The listing builds one solid part. Answer for the finished solid, in the listing's coordinates (mm). A direction names the side the tool comes from. Give positions to 0.01 mm unless a question says otherwise; leave off trailing zeros. Order: outer loops, then holes, each group sorted by start corner. A loop starts at its lowest first (then second) coordinate and runs counter-clockwise, first axis right, second up. Notation, with made-up numbers: (-15.5, -26) -> (-2.5, -26) arc R29 cw to (-2.5, -3) -> close; hole circle Ø9 at (64.5, 48). An arc over 180 degrees is marked (long way). One line per question, with ' | ' between items. Start each with the question number.
Autodesk Inventor part; units mm, degrees
ref_plane "YZ Plane" through (0, 0, 0) normal (1, 0, 0) x (0, 1, 0)
ref_plane "XZ Plane" through (0, 0, 0) normal (0, 1, 0) x (-1, 0, 0)
ref_plane "XY Plane" through (0, 0, 0) normal (0, 0, 1) x (1, 0, 0)
sketch "Esquisse1" plane through (0, 0, 0) normal (0, 1, 0) x (-1, 0, 0)
  circle A0 centre (0, 0) radius 9
  dimension "d0" = 18
extrude "Extrusion1" add sketch "Esquisse1" along normal blind 1
sketch "Esquisse2" plane through (0, 1, 0) normal (0, 1, 0) x (1, 0, 0)
  circle A0 centre (0, 0) radius 9
  circle A1 centre (0, 0) radius 4
  dimension "d3" = 8
extrude "Extrusion2" add sketch "Esquisse2" along normal blind 13 contours A1
sketch "Esquisse3" plane through (0, 14, 0) normal (0, 1, 0) x (1, 0, 0)
  circle A0 centre (0, 0) radius 4
  arc A1 (-2.25, 1.0897) -> (2.25, 1.0897) centre (0, 0) ccw
  line L0 (-2.25, 1.0897) -> (2.25, 1.0897)
  arc A2 (2.25, 1.0897) -> (-2.25, 1.0897) centre (0, 0) ccw
  dimension "d6" = 5
  dimension "d10" = 4.5
extrude "Extrusion3" cut sketch "Esquisse3" against normal through all contours L0 A1
sketch "Esquisse4" plane through (-2.25, 14, -1.0897) normal (0, 0, 1) x (1, 0, 0)
  line L0 (0, 0) -> (4.5, 0)
  line L1 (2.25, -14) -> (2.25, 0) construction
  circle A0 centre (2.25, -10) radius 1.5
  dimension "d11" = 4
  dimension "d12" = 3
extrude "Extrusion4" cut sketch "Esquisse4" against normal up to next
sketch "Esquisse5" plane through (0, 1, 0) normal (0, 1, 0) x (1, 0, 0)
  circle A0 centre (0, 0) radius 4
  circle A1 centre (0, 0) radius 9
  line L0 (0, 0) -> (0, 9) construction
  circle A2 centre (0, 6.5) radius 1.2128
  dimension "d15" = 2.4255
  dimension "d16" = 6.5
extrude "Extrusion5" cut sketch "Esquisse5" against normal up to next contours A2
pattern_circular "Réseau circulaire1" count 6 over 360 about axis through (0, -10, 0) along (0, 1, 0) of "Extrusion5"
thread "Filetage1"
properties part number "axe_roue_moteur"
(1) The part is cut by section A-A on z = 0. Determine the outline of the cut face in (x, y), plus the area to 3 significant figures.
(2) Given P1, Ø3, axis at x = 2, y = 3.5, coming from the -Z side; P2, Ø4, axis at y = 8.5, z = -1.5, coming from the -X side; P3, Ø4, axis at y = 9.5, z = 3, coming from the -X side; P4, Ø1.5, axis at x = -5.63, z = 3.25, coming from the +Y side, each flat-ended and moving along its own axis, determine where each tip first touches the part or whether it passes through.
(3) The part is cut by section D-D on x = 6. Determine the outline of the cut face in (y, z).
(4) For faces 1 (the face through (-1.5, 4.07, -2.52)), 2 (the face through (0, 7, -1.09)), 3 (the face through (-2, 1, -4)), determine the directions among +Z, -Z, +X, -X, +Y, -Y from which every point of the face is accessible in a straight line to the end or side of a thin tool.
(5) The part is cut by section B-B on z = -3.25. Determine the outline of the cut face in (x, y), plus the area to 3 significant figures.
(6) Consider line 1 (Z direction, x = 0, y = 0.5); line 2 (Z direction, x = 0, y = 8); line 3 (Y direction, x = 4.25, z = 7). Determine where each line is inside the solid, lowest interval first.
(7) Determine the mould class of faces 4 (the face through (2.15, 7.409, 3.373)), 5 (the face through (0.263, 0.507, 5.316)), 6 (the face through (0, 14, -2)) for opening direction Z: pulls with the +Z half, pulls with the -Z half, needs draft (parallel to the pull), parting line crosses it, or undercut.
(8) The part is cut by section C-C on z = 3.25. Determine the outline of the cut face in (x, y).
Result sheet:
1) outline: (-9, 0) -> (-2.5, 0) -> (-2.5, 14) -> (-4, 14) -> (-4, 1) -> (-9, 1) -> close; (2.5, 0) -> (9, 0) -> (9, 1) -> (4, 1) -> (4, 14) -> (2.5, 14) -> close | area: 52.0 mm^2
2) P1: stops at z = -3.93 | P2: stops at x = -4 | P3: stops at x = -3.87 | P4: passes through
3) outline: (0, -6.71) -> (1, -6.71) -> (1, -4.4) -> (0, -4.4) -> close; (0, -2.1) -> (1, -2.1) -> (1, 2.1) -> (0, 2.1) -> close; (0, 4.4) -> (1, 4.4) -> (1, 6.71) -> (0, 6.71) -> close
4) face 1: -Z | face 2: +Y, -Y | face 3: +Y
5) outline: (-8.39, 0) -> (-6.84, 0) -> (-6.84, 1) -> (-8.39, 1) -> close; (-4.42, 0) -> (4.42, 0) -> (4.42, 1) -> (2.33, 1) -> (2.33, 14) -> (-2.33, 14) -> (-2.33, 1) -> (-4.42, 1) -> close; (6.84, 0) -> (8.39, 0) -> (8.39, 1) -> (6.84, 1) -> close; hole circle Ø3 at (0, 4) | area: 65.5 mm^2
6) line 1: z = -9 to -7.71, -5.29 to -1.09, 2.5 to 5.29, 7.71 to 9 | line 2: z = -4 to -1.09, 2.5 to 4 | line 3: y = 0 to 1
7) face 4: parting line crosses it | face 5: undercut | face 6: needs draft
8) outline: (-8.39, 0) -> (-6.84, 0) -> (-6.84, 1) -> (-8.39, 1) -> close; (-4.42, 0) -> (4.42, 0) -> (4.42, 1) -> (2.33, 1) -> (2.33, 14) -> (-2.33, 14) -> (-2.33, 1) -> (-4.42, 1) -> close; (6.84, 0) -> (8.39, 0) -> (8.39, 1) -> (6.84, 1) -> close
